from build123d import *

# Parameters (mm, degrees)
SCHNITT_LINEAR_AUSTRAGEN1_DEPTH = 3.5
FASE1_SIZE                      = 0.2
VERRUNDUNG1_R                   = 0.2


with BuildPart() as part:
    # Skizze1 → Rotation1 (revolve)
    with BuildSketch(Plane(origin=(0, 0, 0), x_dir=(0, 0, -1), z_dir=(1, 0, 0)), mode=Mode.PRIVATE) as rotation1_sk:
        with BuildLine():
            Line((-2, 6.9), (0, 6.9))
            Line((0, 6.9), (0, 4))
            Line((0, 4), (18, 4))
            Line((18, 4), (18, 0))
            Line((18, 0), (-6, 0))
            ThreePointArc((-6, 0), (-4.927694437, 3.987793876), (-2, 6.9))
        make_face()
    revolve(rotation1_sk.sketch.rotate(Axis((0, 0, 21.919879518), (0, 0, -1)), 90), axis=Axis((0, 0, 21.919879518), (0, 0, -1)))

    # Skizze2 → Schnitt-Linear austragen1 (cut)
    with BuildSketch(Plane.XY.offset(6)):
        Polygon((2.5, -1.443375673), (2.5, 1.443375673), (0, 2.886751346), (-2.5, 1.443375673), (-2.5, -1.443375673), (0, -2.886751346), align=None)
    extrude(amount=-SCHNITT_LINEAR_AUSTRAGEN1_DEPTH, mode=Mode.SUBTRACT)

    # Fase1
    fase1_edges = [part.edges().sort_by_distance(p)[0] for p in [
        (-6.9, 0, 0),
        (-4, 0, -18),
    ]]
    chamfer(fase1_edges, length=FASE1_SIZE)

    # Verrundung1
    verrundung1_edges = [part.edges().sort_by_distance(p)[0] for p in [
        (2.5, -0.725040561, 5.561851407),
        (1.25, 2.165063509, 5.596754807),
        (-1.25, 2.165063509, 5.596754807),
        (-2.5, 0, 5.596754807),
        (-1.25, -2.165063509, 5.596754807),
        (1.25, -2.165063509, 5.596754807),
        (2.5, -1.443375673, 3.978732003),
        (1.25, -2.165063509, 2.5),
        (0, -2.886751346, 3.978732003),
        (-1.25, -2.165063509, 2.5),
        (-2.5, -1.443375673, 3.978732003),
        (-2.5, 0, 2.5),
        (-2.5, 1.443375673, 3.978732003),
        (-1.25, 2.165063509, 2.5),
        (0, 2.886751346, 3.978732003),
        (1.25, 2.165063509, 2.5),
        (2.5, 1.443375673, 3.978732003),
        (2.5, 0, 2.5),
        (-4, 0, 0),
    ]]
    fillet(verrundung1_edges, radius=VERRUNDUNG1_R)


solid = part.part
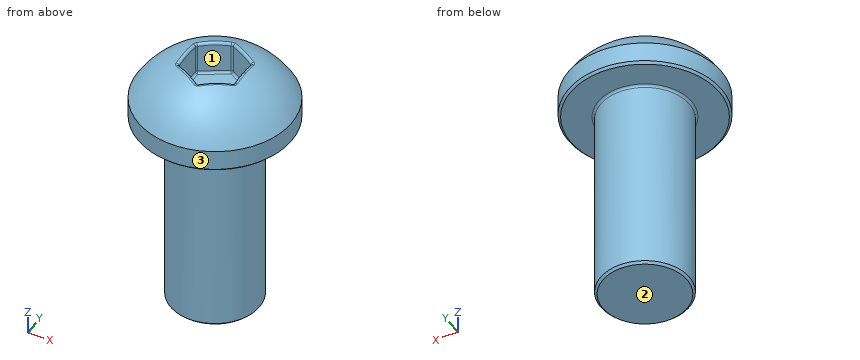
Design review of the part built by this model. Coordinates are the model's own, in mm. Face numbers are marked on the shaded views. Give positions to 0.01 mm unless a question says otherwise; leave off trailing zeros. Loops run counter-clockwise (first coordinate to the right, second up) from the corner with the lowest first, then second, coordinate; pieces in that order, holes last. Notation, with made-up numbers: (80, 86.25) - (111, 86.25) arc R21 cw to (111, 106.25) - close; hole circle Ø4 at (83.5, 34.5). An arc over 180 degrees is marked (long way). Use CSV: the item, a comma, the result in double quotes. Start each with the question number.
1. Add section A-A (z = 3.75). State the section outline as (x, y) points, plus the area to 3 significant figures.
2. Wall thickness on L1, parallel to Z at x = 0.5, y = -2.25; L2, parallel to Z at x = 3, y = 0.5; L3, parallel to X at y = 0.75, z = -4: over which ranges is each line inside the solid? List them lowest first.
3. Draft analysis for pull direction Y (two halves, no side actions). For the marked faces 1, 2 and 3, state which applies: released by +Y, released by -Y, zero draft, split by the parting line, or undercut.
4. Add section B-B (z = -5). State the section outline as (x, y) points, plus the area to 3 significant figures.
5. Insertion check: P1, Ø6, axis at x = 4.5, y = 3, coming from the -Z side; P2, Ø3, axis at y = 0, z = 4, coming from the +X side; P3, Ø3, axis at y = 0.5, z = 4.5, coming from the -X side; P4, Ø1.5, axis at y = 2, z = -3, coming from the -X side. Each pin has a flat end and moves straight along its axis. Give the tip position at first contact, or say it passes through.
Results found:
1,outline,"circle Ø11.08 at (0, 0); hole (-2.5, -1.33) arc R0.2 ccw to (-2.4, -1.5) - (-0.1, -2.83) arc R0.2 ccw to (0.1, -2.83) - (2.4, -1.5) arc R0.2 ccw to (2.5, -1.33) - (2.5, 1.33) arc R0.2 ccw to (2.4, 1.5) - (0.1, 2.83) arc R0.2 ccw to (-0.1, 2.83) - (-2.4, 1.5) arc R0.2 ccw to (-2.5, 1.33) - close"
1,area,"74.9 mm²"
2,L1,"z = -18 to 2.5"
2,L2,"z = -18 to 5.4"
2,L3,"x = -3.93 to 3.93"
3,face 1,"undercut"
3,face 2,"zero draft"
3,face 3,"split by the parting line"
4,outline,"circle Ø8 at (0, 0)"
4,area,"50.3 mm²"
5,P1,"stops at z = -18"
5,P2,"stops at x = 6.59"
5,P3,"stops at x = -6.21"
5,P4,"stops at x = -3.8"
